Geometry check sheet. Reference: the model listing, model coordinates, mm. A direction names the side the tool comes from. Give positions to 0.01 mm unless a question says otherwise; leave off trailing zeros. Loops run counter-clockwise (first coordinate to the right, second up) from the corner with the lowest first, then second, coordinate; pieces in that order, holes last. Notation, with made-up numbers: (-13, -15) - (46, -15) arc R17 cw to (46, 17) - close; hole circle Ø5 at (65.25, 21). An arc over 180 degrees is marked (long way). Use a Markdown table: item, result. Add a question column.
1. Draft check along Y on faces 4 (the flat face through (0, 4, 0)), 5 (the flat face through (0, -16.51, 13)), 6 (the flat face through (-15.494, 0, 11)), 7 (the flat face through (0, 16.51, 13)). Enter one of: pulls with the +Y half, pulls with the -Y half, needs draft (parallel to the pull), parting line crosses it, or undercut.
2. Cross-section at C-C on x = 0. Enter the section's corners in (y, z).
3. Depth check by flat-ended pin: P1, Ø13.5, axis at x = 0, y = 2, coming from the +Z side; P2, Ø0.9, axis at x = 15, y = 0.5, coming from the -Z side; P3, Ø4, axis at x = 0, y = 0, coming from the +Z side. Enter the tip coordinate at first touch or a pass-through.
4. Material ranges on L1, parallel to Y at x = 0, z = 0.7; L2, parallel to X at y = -13.5, z = 17.75; L3, parallel to X at y = 9.5, z = 20, recorded low to high.
5. Set-up check for faces 1 (the cylindrical face through (-0.31, 2.33, 1.25)), 2 (the flat face through (-15, -13.716, 11)), 3 (the flat face through (0, -3, 2.54)): record each of +Z, -Z, +X, -X, +Y, -Y from which the full face is reachable in a straight line by a thin tool's end or side.
6. Cross-section at B-B on z = 10.5. Enter the section's corners in (x, y), and give its area (3 significant figures).
7. Cross-section at D-D on x = 15. Enter the section's corners in (y, z), and give its area (3 significant figures).
8. Cross-section at A-A on y = 0. Enter the section's corners in (x, z), and give its area (3 significant figures).
from build123d import *

# Parameters (mm, degrees)
F0_W     = 38.1
F0_H     = 33.02
F0_R     = 2.3495
F1_DEPTH = 2.54
F2_W     = 38.1
F2_H     = 33.02
F2_R     = 13.462
F3_DEPTH = 22.86
F4_W     = 1.778
F4_H     = 27.432
F5_DEPTH = 21.59


with BuildPart() as f1:
    # F0 (on Top) → F1 (new body)
    with BuildSketch(Plane.XY):
        Rectangle(F0_W, F0_H)
        Circle(F0_R, mode=Mode.SUBTRACT)
    extrude(amount=F1_DEPTH)

    # F2 (on face) → F3 (join)
    with BuildSketch(Plane.XY.offset(2.54)):
        Rectangle(F2_W, F2_H)
        Circle(F2_R, mode=Mode.SUBTRACT)
    extrude(amount=F3_DEPTH)

    # F4 (on face) → F5 (cut)
    with BuildSketch(Plane(origin=(0, 0, 0), x_dir=(1, 0, 0), z_dir=(0, 0, -1))):
        with Locations((14.605, 0)):
            Rectangle(F4_W, F4_H)
        with Locations((-14.605, 0)):
            Rectangle(F4_W, F4_H)
    extrude(amount=-F5_DEPTH, mode=Mode.SUBTRACT)


solid = f1.part
Values found:
| question | item | result |
|---|---|---|
| 1 | face 4 | needs draft |
| 1 | face 5 | pulls with the -Y half |
| 1 | face 6 | undercut |
| 1 | face 7 | pulls with the +Y half |
| 2 | outline | (-16.51, 0) - (-2.35, 0) - (-2.35, 2.54) - (-13.46, 2.54) - (-13.46, 25.4) - (-16.51, 25.4) - close; (2.35, 0) - (16.51, 0) - (16.51, 25.4) - (13.46, 25.4) - (13.46, 2.54) - (2.35, 2.54) - close |
| 3 | P1 | stops at z = 2.54 |
| 3 | P2 | stops at z = 21.59 |
| 3 | P3 | passes through |
| 4 | L1 | y = -16.51 to -2.35, 2.35 to 16.51 |
| 4 | L2 | x = -19.05 to -15.49, -13.72 to 13.72, 15.49 to 19.05 |
| 4 | L3 | x = -19.05 to -15.49, -13.72 to -9.54, 9.54 to 13.72, 15.49 to 19.05 |
| 5 | face 1 | +Z, -Z |
| 5 | face 2 | -Z |
| 5 | face 3 | +Z |
| 6 | outline | (-19.05, -16.51) - (19.05, -16.51) - (19.05, 16.51) - (-19.05, 16.51) - close; hole (-15.49, -13.72) - (-13.72, -13.72) - (-13.72, 13.72) - (-15.49, 13.72) - close; hole circle Ø26.92 at (0, 0); hole (13.72, -13.72) - (15.49, -13.72) - (15.49, 13.72) - (13.72, 13.72) - close |
| 6 | area | 591 mm2 |
| 7 | outline | (-16.51, 0) - (-13.72, 0) - (-13.72, 21.59) - (13.72, 21.59) - (13.72, 0) - (16.51, 0) - (16.51, 25.4) - (-16.51, 25.4) - close |
| 7 | area | 246 mm2 |
| 8 | outline | (-19.05, 0) - (-15.49, 0) - (-15.49, 21.59) - (-13.72, 21.59) - (-13.72, 0) - (-2.35, 0) - (-2.35, 2.54) - (-13.46, 2.54) - (-13.46, 25.4) - (-19.05, 25.4) - close; (2.35, 0) - (13.72, 0) - (13.72, 21.59) - (15.49, 21.59) - (15.49, 0) - (19.05, 0) - (19.05, 25.4) - (13.46, 25.4) - (13.46, 2.54) - (2.35, 2.54) - close |
| 8 | area | 264 mm2 |
